```python
from build123d import *

# Parameters (mm, degrees)
SKETCH_W        = 81.25
SKETCH_H        = 81.25
SKETCH_W_2      = 14
SKETCH_H_2      = 14
PAD_DEPTH       = 1.5
SKETCH001_W     = 81.25
SKETCH001_H     = 81.25
SKETCH001_W_2   = 76.25
SKETCH001_H_2   = 76.25
PAD001_DEPTH    = 14
FILLET_R        = 5.05
FILLET001_R     = 2.5
SKETCH002_W     = 2
SKETCH002_H     = 4
POCKET_DEPTH    = 85
SKETCH003_W     = 2
SKETCH003_H     = 4
POCKET001_DEPTH = 86


with BuildPart() as part:
    # Sketch → Pad (new body)
    with BuildSketch(Plane.XY):
        with Locations((40.625, 40.625)):
            Rectangle(SKETCH_W, SKETCH_H)
        with Locations((12.05, 69.2)):
            Rectangle(SKETCH_W_2, SKETCH_H_2, mode=Mode.SUBTRACT)
        with Locations((31.1, 69.2)):
            Rectangle(SKETCH_W_2, SKETCH_H_2, mode=Mode.SUBTRACT)
        with Locations((50.15, 69.2)):
            Rectangle(SKETCH_W_2, SKETCH_H_2, mode=Mode.SUBTRACT)
        with Locations((69.2, 69.2)):
            Rectangle(SKETCH_W_2, SKETCH_H_2, mode=Mode.SUBTRACT)
        with Locations((12.05, 50.15)):
            Rectangle(SKETCH_W_2, SKETCH_H_2, mode=Mode.SUBTRACT)
        with Locations((31.1, 50.15)):
            Rectangle(SKETCH_W_2, SKETCH_H_2, mode=Mode.SUBTRACT)
        with Locations((50.15, 50.15)):
            Rectangle(SKETCH_W_2, SKETCH_H_2, mode=Mode.SUBTRACT)
        with Locations((69.2, 50.15)):
            Rectangle(SKETCH_W_2, SKETCH_H_2, mode=Mode.SUBTRACT)
        with Locations((12.05, 31.1)):
            Rectangle(SKETCH_W_2, SKETCH_H_2, mode=Mode.SUBTRACT)
        with Locations((31.1, 31.1)):
            Rectangle(SKETCH_W_2, SKETCH_H_2, mode=Mode.SUBTRACT)
        with Locations((50.15, 31.1)):
            Rectangle(SKETCH_W_2, SKETCH_H_2, mode=Mode.SUBTRACT)
        with Locations((69.2, 31.1)):
            Rectangle(SKETCH_W_2, SKETCH_H_2, mode=Mode.SUBTRACT)
        with Locations((12.05, 12.05)):
            Rectangle(SKETCH_W_2, SKETCH_H_2, mode=Mode.SUBTRACT)
        with Locations((31.1, 12.05)):
            Rectangle(SKETCH_W_2, SKETCH_H_2, mode=Mode.SUBTRACT)
        with Locations((50.15, 12.05)):
            Rectangle(SKETCH_W_2, SKETCH_H_2, mode=Mode.SUBTRACT)
        with Locations((69.2, 12.05)):
            Rectangle(SKETCH_W_2, SKETCH_H_2, mode=Mode.SUBTRACT)
    extrude(amount=PAD_DEPTH)

    # Sketch001 (on Face70 of Pad) → Pad001 (join)
    with BuildSketch(Plane.XY.offset(1.5)):
        with Locations((40.625, 40.625)):
            Rectangle(SKETCH001_W, SKETCH001_H)
        with Locations((40.625, 40.625)):
            Rectangle(SKETCH001_W_2, SKETCH001_H_2, mode=Mode.SUBTRACT)
    extrude(amount=PAD001_DEPTH)

    # Fillet
    fillet_edges = [part.edges().sort_by_distance(p)[0] for p in [
        (0, 0, 8.5),
        (81.25, 0, 8.5),
        (81.25, 81.25, 8.5),
        (0, 81.25, 8.5),
    ]]
    fillet(fillet_edges, radius=FILLET_R)

    # Fillet001
    fillet001_edges = [part.edges().sort_by_distance(p)[0] for p in [
        (2.5, 78.75, 8.5),
        (2.5, 2.5, 8.5),
        (78.75, 2.5, 8.5),
        (78.75, 78.75, 8.5),
    ]]
    fillet(fillet001_edges, radius=FILLET001_R)

    # Sketch002 (on Face10 of Fillet001) → Pocket (cut)
    with BuildSketch(Plane.XZ):
        with Locations((40.625, 13.5)):
            Rectangle(SKETCH002_W, SKETCH002_H)
        with Locations((21.575, 13.5)):
            Rectangle(SKETCH002_W, SKETCH002_H)
        with Locations((59.675, 13.5)):
            Rectangle(SKETCH002_W, SKETCH002_H)
    extrude(amount=-POCKET_DEPTH, mode=Mode.SUBTRACT)

    # Sketch003 (on Face9 of Pocket) → Pocket001 (cut)
    with BuildSketch(Plane(origin=(0, 0, 0), x_dir=(0, -1, 0), z_dir=(-1, 0, 0))):
        with Locations((-40.625, 13.5)):
            Rectangle(SKETCH003_W, SKETCH003_H)
        with Locations((-21.575, 13.5)):
            Rectangle(SKETCH003_W, SKETCH003_H)
        with Locations((-59.675, 13.5)):
            Rectangle(SKETCH003_W, SKETCH003_H)
    extrude(amount=-POCKET001_DEPTH, mode=Mode.SUBTRACT)


solid = part.part
```
Work out the finished part from the listing and answer in its coordinate system (mm). A direction names the side the tool comes from. Give positions to 0.01 mm unless a question says otherwise; leave off trailing zeros. Write each loop counter-clockwise with the first axis right and the second up, starting at its lowest first coordinate (ties: lowest second). Pieces come first, ordered by that corner, then holes. Notation, with made-up numbers: (84.5, 37.5) -> (96.5, 37.5) arc R13 cw to (96.5, 57.5) -> close; hole circle Ø2 at (23, 86). An arc over 180 degrees is marked (long way). Write each question's results on one line, items separated by ' | '.
1. Each of these flat-tipped pins is pushed along its axis until it touches: pin 1 Ø12 at (x, y) = (13.5, 51) entering from +Z; pin 2 Ø0.6 at (x, y) = (41, 79.5) entering from +Z; pin 3 Ø2 at (x, z) = (1, 14) entering from +Y. Where does it stop, or does it pass through?
Data:
pin 1: z = 1.5 | pin 2: z = 11.5 | pin 3: y = 80.22
2. A tool of negligible diameter and unlimited length cuts with its end or side. For faces 5 (the flat face through (2, 76, 15.5)), 6 (the flat face through (1, 22, 11.5)), 7 (the flat face through (41.625, 1, 13)), 8 (the cylindrical face through (77.998, 3.213, 8.598)), from which of +Z, -Z, +X, -X, +Y, -Y can it reach the whole face along a straight path? Write none if from no direction.
Data:
face 5: +Z, +X, -X, +Y, -Y | face 6: +Z, +X, -X | face 7: +Z, +Y, -Y | face 8: +Z
3. Find section A-A on y = 26.5. Determine the outline of the cut face in (x, z).
Data:
outline: (0, 0) -> (5.05, 0) -> (5.05, 1.5) -> (2.5, 1.5) -> (2.5, 15.5) -> (0, 15.5) -> close; (19.05, 0) -> (24.1, 0) -> (24.1, 1.5) -> (19.05, 1.5) -> close; (38.1, 0) -> (43.15, 0) -> (43.15, 1.5) -> (38.1, 1.5) -> close; (57.15, 0) -> (62.2, 0) -> (62.2, 1.5) -> (57.15, 1.5) -> close; (76.2, 0) -> (81.25, 0) -> (81.25, 15.5) -> (78.75, 15.5) -> (78.75, 1.5) -> (76.2, 1.5) -> close
4. Straight lines are drawn through the part: L1, parallel to Y at x = 76, z = 0.5; L2, parallel to Y at x = 20.5, z = 10.5. For each, find the intervals that lie inside material, in ascending order.
Data:
L1: 0 to 5.05, 19.05 to 24.1, 38.1 to 43.15, 57.15 to 62.2, 76.2 to 81.25 | L2: 0 to 2.5, 78.75 to 81.25
5. Find section D-D on z = 14.25. Give the number of separate pieces and of enclosed holes in the cut face, and give its area (3 significant figures).
Data:
separate pieces: 12 | enclosed holes: 0 | area: 711 mm^2
6. Determine the mould class of faces 1 (the flat face through (40, 81.25, 8)), 2 (the flat face through (40, 0, 8)), 3 (the flat face through (80, 60, 11.5)), 4 (the flat face through (58.675, 80, 13)) for opening direction Y: +Y half, -Y half, draft (parallel to the pull), parting line (faces both ways), or undercut.
Data:
face 1: +Y half | face 2: -Y half | face 3: undercut | face 4: draft
7. Find section C-C on z = 9. Determine the outline of the cut face in (x, y).
Data:
outline: (0, 5.05) arc R5.05 ccw to (5.05, 0) -> (76.2, 0) arc R5.05 ccw to (81.25, 5.05) -> (81.25, 76.2) arc R5.05 ccw to (76.2, 81.25) -> (5.05, 81.25) arc R5.05 ccw to (0, 76.2) -> close; hole (2.5, 5) arc R2.5 ccw to (5, 2.5) -> (76.25, 2.5) arc R2.5 ccw to (78.75, 5) -> (78.75, 76.25) arc R2.5 ccw to (76.25, 78.75) -> (5, 78.75) arc R2.5 ccw to (2.5, 76.25) -> close
